Work out the finished part from the listing and answer in its coordinate system (mm). A direction names the side the tool comes from. Give positions to 0.01 mm unless a question says otherwise; leave off trailing zeros. Write each loop counter-clockwise with the first axis right and the second up, starting at its lowest first coordinate (ties: lowest second). Pieces come first, ordered by that corner, then holes. Notation, with made-up numbers: (67, 17.5) -> (87, 17.5) arc R37 cw to (87, 56.5) -> close; hole circle Ø11 at (-6, 45.25). An arc over 180 degrees is marked (long way). Write item = value, one per line. Start each with the question number.
from build123d import *

# Parameters (mm, degrees)
EXTRUDE_1_DEPTH      = 250
EXTRUDE_1_DEPTH_BACK = 250
SHELL_1_T            = -3
CHAMFER_1_SIZE       = 5.358983849
CHAMFER_1_SIZE_2     = 20


with BuildPart() as part:
    # Эскиз1 → Бобышка-Вытянуть1 (new, two sides: drawn at the far end of the back side and taken through both)
    with BuildSketch(Plane.XY.offset(-EXTRUDE_1_DEPTH_BACK)):
        with BuildLine():
            Line((-14, 10), (14, 10))
            ThreePointArc((14, 10), (18.242640687, 8.242640687), (20, 4))
            Line((20, 4), (20, -4))
            ThreePointArc((20, -4), (18.242640687, -8.242640687), (14, -10))
            Line((14, -10), (-14, -10))
            ThreePointArc((-14, -10), (-18.242640687, -8.242640687), (-20, -4))
            Line((-20, -4), (-20, 4))
            ThreePointArc((-20, 4), (-18.242640687, 8.242640687), (-14, 10))
        make_face()
    extrude(amount=EXTRUDE_1_DEPTH + EXTRUDE_1_DEPTH_BACK)

    # Оболочка1
    shell_1_openings = [part.faces().sort_by_distance(p)[0] for p in [
        (0, 0, -250),
        (0, 0, 250),
    ]]
    offset(amount=SHELL_1_T, openings=shell_1_openings, kind=Kind.INTERSECTION)

    # Фаска1
    # the kernel refuses this chamfer: 20, 5.358983849 mm, written as the material it takes off along each edge
    with BuildSketch(Plane(origin=(-65.934431404, 10, -250), x_dir=(0, 0.1375124470212891, 0.9905000388259543), z_dir=(1, 0, 0))) as chamfer_1_piece_1:
        Polygon((CHAMFER_1_SIZE * 0.990500038756, CHAMFER_1_SIZE * 0.137512447012), (-CHAMFER_1_SIZE_2 * 0.137512447021, CHAMFER_1_SIZE_2 * 0.990500038826), (0, 0), align=None)
    extrude(amount=131.868862808, mode=Mode.SUBTRACT)
    with BuildSketch(Plane(origin=(-65.934431404, 10, 250), x_dir=(0, 0.1375124470212891, -0.9905000388259543), z_dir=(1, 0, 0))) as chamfer_1_piece_2:
        Polygon((CHAMFER_1_SIZE * 0.990500038756, -CHAMFER_1_SIZE * 0.137512447012), (-CHAMFER_1_SIZE_2 * 0.137512447021, -CHAMFER_1_SIZE_2 * 0.990500038826), (0, 0), align=None)
    extrude(amount=131.868862808, mode=Mode.SUBTRACT)


solid = part.part
(1) Determine the mould class of faces 3 (the flat face through (-0.093, 7.454, -245.323)), 4 (the flat face through (0, 10, -3)), 5 (the flat face through (-0.093, 7.454, 245.323)) for opening direction Z: pulls with the +Z half, pulls with the -Z half, needs draft (parallel to the pull), parting line crosses it, or undercut.
(2) Find the intervals of material crossed by line 1 along X through (y, z) = (-3.25, -13.5); line 2 along Y through (x, z) = (-10.5, -64); line 3 along Y through (x, z) = (-15.5, 75), in increasing order.
(3) This flat-tipped pin is pushed along its axis until it touches: pin 1 (2 mm diameter, centred on x = -0.5, y = -7, fed in from -Z). Where does it stop, or does it pass through?
(4) For faces 1 (the flat face through (20, 0, -3)), 2 (the flat face through (17, 0, -3)), determine the directions among +Z, -Z, +X, -X, +Y, -Y from which every point of the face is accessible in a straight line to the end or side of a thin tool.
(5) A cutting plane is placed at B-B, the plane z = 166.5. Write down the section's boundary in (x, y).
(6) A cutting plane is placed at A-A, the plane x = 4. Write down the section's boundary in (y, z), then the cut area to 3 significant figures.
(7) A cutting plane is placed at C-C, the plane y = 0.5. Write down the section's boundary in (x, z).
Results list:
q1.face_3 = pulls with the -Z half
q1.face_4 = needs draft
q1.face_5 = pulls with the +Z half
q2.line_1 = -20 to -17, 17 to 20
q2.line_2 = -10 to -7, 7 to 10
q2.line_3 = -9.81 to -6.6, 6.6 to 9.81
q3.pin_1 = -249.46
q4.face_1 = +Z, -Z, +X, +Y, -Y
q4.face_2 = +Z, -Z
q5.outline = (-20, -4) arc R6 ccw to (-14, -10) -> (14, -10) arc R6 ccw to (20, -4) -> (20, 4) arc R6 ccw to (14, 10) -> (-14, 10) arc R6 ccw to (-20, 4) -> close; hole (-17, -4) arc R3 ccw to (-14, -7) -> (14, -7) arc R3 ccw to (17, -4) -> (17, 4) arc R3 ccw to (14, 7) -> (-14, 7) arc R3 ccw to (-17, 4) -> close
q6.outline = (-10, -250) -> (-7, -249.2) -> (-7, 249.2) -> (-10, 250) -> close; (7, -245.44) -> (10, -244.64) -> (10, 244.64) -> (7, 245.44) -> close
q6.area = 2,970 mm²
q7.outline = (-20, -247.19) -> (-17, -247.19) -> (-17, 247.19) -> (-20, 247.19) -> close; (17, -247.19) -> (20, -247.19) -> (20, 247.19) -> (17, 247.19) -> close
